Design review of the part built by this model. Coordinates are the model's own, in mm. Round coordinates to 2 decimals unless told otherwise and drop trailing zeros. Loops run counter-clockwise (first coordinate to the right, second up) from the corner with the lowest first, then second, coordinate; pieces in that order, holes last. Notation, with made-up numbers: (-2, 77) - (43, 77) arc R32 ccw to (43, 108) - close; hole circle Ø11 at (78, -1). An arc over 180 degrees is marked (long way). Use one line per item in the form item = value. Start each with the question number.
(1) Wall thickness on probe 1 along Z at (x, y) = (-229.5, -1.5); probe 2 along Z at (x, y) = (204, -2.25); probe 3 along X at (y, z) = (-4.25, -100.5): over which ranges is each line inside the solid? List them lowest first. Write a range as [from, to].
(2) We need section D-D, the plane y = 0.5. Give the number of separate pieces and of enclosed holes in the cut face, then the cut area to 3 significant figures.
(3) We need section A-A, the plane x = 169. Write out the cut boundary in (y, z).
(4) We need section B-B, the plane z = -163. Write out the cut boundary in (x, y), then the cut area to 3 significant figures.
(5) For pin 1 (3 mm diameter, centred on y = -1.5, z = -210, fed in from -X); pin 2 (3 mm diameter, centred on x = 282.5, y = -2.5, fed in from -Z); pin 3 (3 mm diameter, centred on x = 283.5, y = -1, fed in from +Z), all flat-tipped, find the tip position at first contact; note any pin that passes through.
(6) We need section C-C, the plane x = -204. Write out the cut boundary in (y, z), then the cut area to 3 significant figures.
from build123d import *

# Parameters (mm, degrees)
SKETCH1_W           = 580
SKETCH1_H           = 430
SKETCH1_W_2         = 130
SKETCH1_H_2         = 60
SKETCH1_W_3         = 35
SKETCH1_H_3         = 44
BOSS_EXTRUDE1_DEPTH = 5
SKETCH2_W           = 20
SKETCH2_H           = 20
CUT_EXTRUDE1_DEPTH  = 10
SKETCH3_W           = 130
SKETCH3_H           = 60
SKETCH3_W_2         = 35
SKETCH3_H_2         = 44
CUT_EXTRUDE2_DEPTH  = 98
SKETCH4_W           = 20
SKETCH4_H           = 20
CUT_EXTRUDE3_DEPTH  = 98


with BuildPart() as part:
    # Sketch1 → Boss-Extrude1 (new, symmetric)
    with BuildSketch(Plane(origin=(0, 0, 0), x_dir=(1, 0, 0), z_dir=(0, 1, 0))):
        Rectangle(SKETCH1_W, SKETCH1_H)
        with Locations((-193.023255814, 165)):
            Rectangle(SKETCH1_W_2, SKETCH1_H_2, mode=Mode.SUBTRACT)
        with Locations((-193.023255814, -165)):
            Rectangle(SKETCH1_W_2, SKETCH1_H_2, mode=Mode.SUBTRACT)
        with Locations((-193.023255814, -85)):
            Rectangle(SKETCH1_W_3, SKETCH1_H_3, mode=Mode.SUBTRACT)
        with Locations((-193.023255814, 85)):
            Rectangle(SKETCH1_W_3, SKETCH1_H_3, mode=Mode.SUBTRACT)
    extrude(amount=BOSS_EXTRUDE1_DEPTH, both=True)

    # Sketch2 → Cut-Extrude1 (cut)
    with BuildSketch(Plane(origin=(0, 5, 0), x_dir=(1, 0, 0), z_dir=(0, 1, 0))):
        with Locations((-280, 205)):
            Rectangle(SKETCH2_W, SKETCH2_H)
        with Locations((280, 205)):
            Rectangle(SKETCH2_W, SKETCH2_H)
        with Locations((280, -205)):
            Rectangle(SKETCH2_W, SKETCH2_H)
        with Locations((-280, -205)):
            Rectangle(SKETCH2_W, SKETCH2_H)
    extrude(amount=-CUT_EXTRUDE1_DEPTH, mode=Mode.SUBTRACT)

    # Sketch3 → Cut-Extrude2 (cut)
    with BuildSketch(Plane(origin=(0, 5, 0), x_dir=(1, 0, 0), z_dir=(0, 1, 0))):
        with Locations((193.023255814, -165)):
            Rectangle(SKETCH3_W, SKETCH3_H)
        with Locations((-193.023255814, 165)):
            Rectangle(SKETCH3_W, SKETCH3_H)
        with Locations((193.023255814, -85)):
            Rectangle(SKETCH3_W_2, SKETCH3_H_2)
        with Locations((-193.023255814, 85)):
            Rectangle(SKETCH3_W_2, SKETCH3_H_2)
        with Locations((-193.023255814, -85)):
            Rectangle(SKETCH3_W_2, SKETCH3_H_2)
        with Locations((-193.023255814, -165)):
            Rectangle(SKETCH3_W, SKETCH3_H)
        with Locations((193.023255814, 85)):
            Rectangle(SKETCH3_W_2, SKETCH3_H_2)
        with Locations((193.023255814, 165)):
            Rectangle(SKETCH3_W, SKETCH3_H)
    extrude(amount=-CUT_EXTRUDE2_DEPTH, mode=Mode.SUBTRACT)

    # Sketch4 → Cut-Extrude3 (cut)
    with BuildSketch(Plane(origin=(0, 5, 0), x_dir=(1, 0, 0), z_dir=(0, 1, 0))):
        with Locations((-20, -205)):
            Rectangle(SKETCH4_W, SKETCH4_H)
        with Locations((-20, 205)):
            Rectangle(SKETCH4_W, SKETCH4_H)
    extrude(amount=-CUT_EXTRUDE3_DEPTH, mode=Mode.SUBTRACT)


solid = part.part
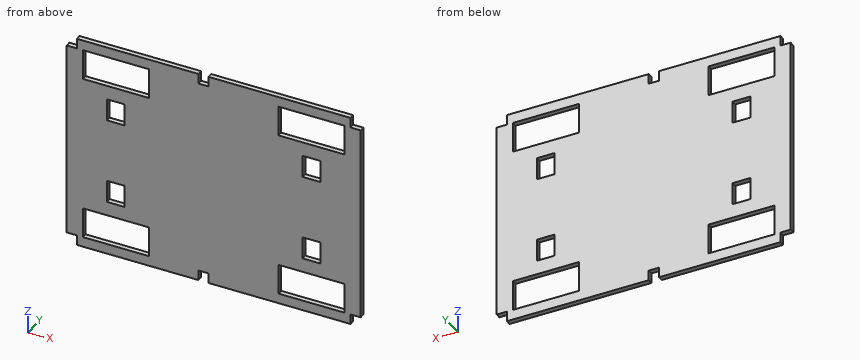
Data:
q1.probe_1 = [-215, -195], [-135, 135], [195, 215]
q1.probe_2 = [-215, -195], [-135, -107], [-63, 63], [107, 135], [195, 215]
q1.probe_3 = [-290, -210.52], [-175.52, 175.52], [210.52, 290]
q2.separate_pieces = 1
q2.enclosed_holes = 8
q2.area = 210,000 mm^2
q3.outline = (-5, -215) - (5, -215) - (5, -195) - (-5, -195) - close; (-5, -135) - (5, -135) - (5, 135) - (-5, 135) - close; (-5, 195) - (5, 195) - (5, 215) - (-5, 215) - close
q4.outline = (-290, -5) - (-258.02, -5) - (-258.02, 5) - (-290, 5) - close; (-128.02, -5) - (128.02, -5) - (128.02, 5) - (-128.02, 5) - close; (258.02, -5) - (290, -5) - (290, 5) - (258.02, 5) - close
q4.area = 3,200 mm^2
q5.pin_1 = -270
q5.pin_2 = -195
q5.pin_3 = 195
q6.outline = (-5, -215) - (5, -215) - (5, -195) - (-5, -195) - close; (-5, -135) - (5, -135) - (5, -107) - (-5, -107) - close; (-5, -63) - (5, -63) - (5, 63) - (-5, 63) - close; (-5, 107) - (5, 107) - (5, 135) - (-5, 135) - close; (-5, 195) - (5, 195) - (5, 215) - (-5, 215) - close
q6.area = 2,220 mm^2
